Answer from the drawing. Dimensions are ordinates in mm from the lowest x, y and z of the part. Coordinates: 2 decimals unless noted, no trailing zeros. Write each loop counter-clockwise with the first axis right and the second up, starting at its lowest first coordinate (ties: lowest second). Pieces come first, ordered by that corner, then holes.
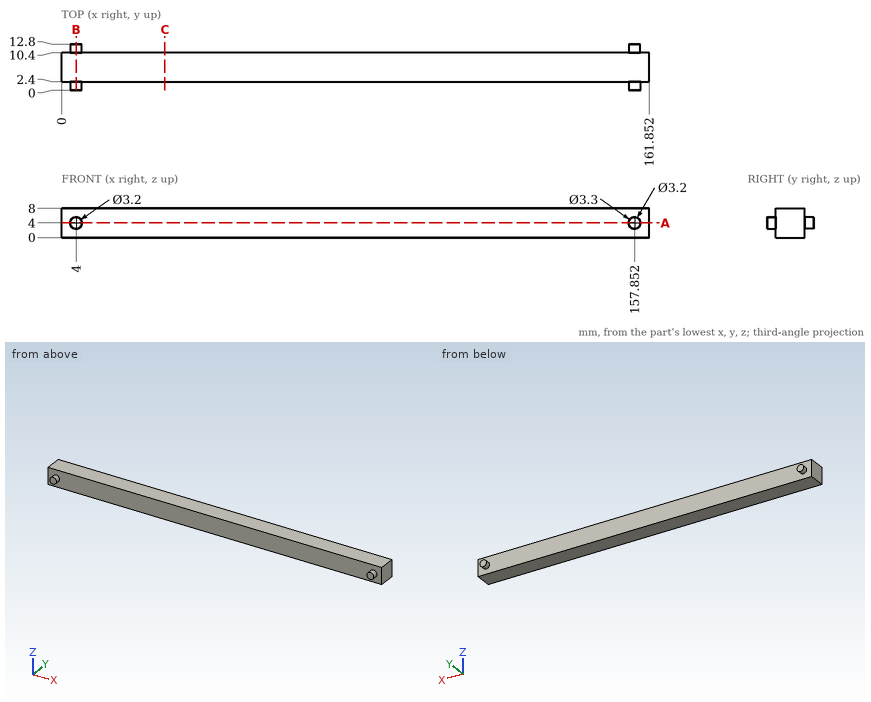
(1) Find the intervals of material crossed by probe 1 along Y at (x, z) = (58, 3.25), in increasing order.
(2) Section B-B, the plane x = 4 is taken. Write down the section's boundary in (y, z).
(3) Each of these flat-tipped pins is pushed along its axis until it touches: pin 1 (4 mm diameter, centred on x = 73, z = 1, fed in from -Y); pin 2 (1 mm diameter, centred on x = 144.5, z = 5.5, fed in from +Y). Where does it stop, or does it pass through?
(4) Section C-C, the plane x = 28.5 is taken. Write down the section's boundary in (y, z), plus the area to 3 significant figures.
(5) Section A-A, the plane z = 4 is taken. Write down the section's boundary in (x, y), plus the area to 3 significant figures.
Solution:
1. probe 1: y = 2.4 to 10.4
2. outline: (0, 2.4) - (2.4, 2.4) - (2.4, 0) - (10.4, 0) - (10.4, 2.4) - (12.8, 2.4) - (12.8, 5.6) - (10.4, 5.6) - (10.4, 8) - (2.4, 8) - (2.4, 5.6) - (0, 5.6) - close
3. pin 1: stops at y = 2.4
3. pin 2: stops at y = 10.4
4. outline: (2.4, 0) - (10.4, 0) - (10.4, 8) - (2.4, 8) - close
4. area: 64.0 mm2
5. outline: (0, 2.4) - (2.4, 2.4) - (2.4, 0) - (5.6, 0) - (5.6, 2.4) - (156.2, 2.4) - (156.2, 0) - (159.5, 0) - (159.5, 2.4) - (161.85, 2.4) - (161.85, 10.4) - (159.45, 10.4) - (159.45, 12.8) - (156.25, 12.8) - (156.25, 10.4) - (5.6, 10.4) - (5.6, 12.8) - (2.4, 12.8) - (2.4, 10.4) - (0, 10.4) - close
5. area: 1,330 mm2
